from build123d import *

# Parameters (mm, degrees)
BOSS_EXTRUDE1_DEPTH = 1.5875
SKETCH2_W           = 4.5
SKETCH2_H           = 3.5
CUT_EXTRUDE1_DEPTH  = 2.5875
CHAMFER1_SIZE       = 1


with BuildPart() as part:
    # Sketch1 → Boss-Extrude1 (new body)
    with BuildSketch(Plane.XY):
        with BuildLine():
            Line((4.207, 4.461), (-4.207, 4.461))
            ThreePointArc((-4.207, 4.461), (-4.386605122, 4.386605122), (-4.461, 4.207))
            Line((-4.461, 4.207), (-4.461, -4.207))
            ThreePointArc((-4.461, -4.207), (-4.386605122, -4.386605122), (-4.207, -4.461))
            Line((-4.207, -4.461), (4.207, -4.461))
            ThreePointArc((4.207, -4.461), (4.386605122, -4.386605122), (4.461, -4.207))
            Line((4.461, -4.207), (4.461, 4.207))
            ThreePointArc((4.461, 4.207), (4.386605122, 4.386605122), (4.207, 4.461))
        make_face()
    extrude(amount=BOSS_EXTRUDE1_DEPTH)

    # Sketch2 → Cut-Extrude1 (cut, through all)
    with BuildSketch(Plane.XY.offset(1.5875)):
        Rectangle(SKETCH2_W, SKETCH2_H)
    extrude(amount=-CUT_EXTRUDE1_DEPTH, mode=Mode.SUBTRACT)

    # Chamfer1
    chamfer1_edges = [part.edges().sort_by_distance(p)[0] for p in [
        (2.25, 1.75, 0.79375),
        (2.25, -1.75, 0.79375),
        (-2.25, -1.75, 0.79375),
        (-2.25, 1.75, 0.79375),
    ]]
    chamfer(chamfer1_edges, length=CHAMFER1_SIZE)


solid = part.part
Build history of the part. All positions in model axes, mm. A direction names the side the tool comes from. Coordinates: 2 decimals unless noted, no trailing zeros. Order: outer loops, then holes, each group sorted by start corner. A loop starts at its lowest first (then second) coordinate and runs counter-clockwise, first axis right, second up. Notation, with made-up numbers: (-38.75, -10.5) - (-22.75, -10.5) arc R23 ccw to (-22.75, 19.5) - close; hole circle Ø2 at (24, -35.75). An arc over 180 degrees is marked (long way). Write item = value, one per line. Start each with the question number.
1) Saw through at A-A on y = 1. Write the cut outline in (x, z).
2) Saw through at B-B on x = -1.5. Write the cut outline in (y, z), then the cut area to 3 significant figures.
3) Two-plate mould, pull along Y, no slides. Class faces 1 (the face through (2, 1, 1)), 2 (the face through (0, -4.461, 1)), 3 (the face through (4.461, 0, 1)): pulls with the +Y half, pulls with the -Y half, needs draft (parallel to the pull), parting line crosses it, or undercut.
4) Saw through at C-C on z = 0.6. Write the cut outline in (x, y).
5) Wall check: line 1 along X through (y, z) = (-1.25, 0.65); line 2 along X through (y, z) = (-0.5, 0.1). Give the ranges that are in metal, low to high. Write a range as from..to.
6) Flat gauge pin, fed straight in: pin 1 Ø1 at (x, y) = (-3, 3) entering from -Z. Where does the tip first touch, or does it go through?
7) 3-axis set-ups, long thin cutter, end or side, ignore diameter. For faces 4 (the face through (-2, -1, 1)), 5 (the face through (0, 4.461, 1)): which of +Z, -Z, +X, -X, +Y, -Y reach the whole face in a straight line?
From the geometry:
q1.outline = (-4.46, 0) - (-2, 0) - (-2, 1.59) - (-4.46, 1.59) - close; (2, 0) - (4.46, 0) - (4.46, 1.59) - (2, 1.59) - close
q2.outline = (-4.46, 0) - (-1.5, 0) - (-1.5, 1.59) - (-4.46, 1.59) - close; (1.5, 0) - (4.46, 0) - (4.46, 1.59) - (1.5, 1.59) - close
q2.area = 9.40 mm^2
q3.face_1 = undercut
q3.face_2 = pulls with the -Y half
q3.face_3 = needs draft
q4.outline = (-4.46, -4.21) arc R0.25 ccw to (-4.21, -4.46) - (4.21, -4.46) arc R0.25 ccw to (4.46, -4.21) - (4.46, 4.21) arc R0.25 ccw to (4.21, 4.46) - (-4.21, 4.46) arc R0.25 ccw to (-4.46, 4.21) - close; hole (-2.25, -0.75) - (-1.25, -1.75) - (1.25, -1.75) - (2.25, -0.75) - (2.25, 0.75) - (1.25, 1.75) - (-1.25, 1.75) - (-2.25, 0.75) - close
q5.line_1 = -4.46..-1.75, 1.75..4.46
q5.line_2 = -4.46..-2.25, 2.25..4.46
q6.pin_1 = 0
q7.face_4 = +Z, -Z
q7.face_5 = +Z, -Z, +X, -X, +Y
